```python
from build123d import *

# Parameters (mm, degrees)
AUFSATZ_LINEAR_AUSTRAGEN1_DEPTH = 5
SKIZZE2_W                       = 6
SKIZZE2_H                       = 10
AUFSATZ_LINEAR_AUSTRAGEN2_DEPTH = 10
FASE1_SIZE                      = 10
SKIZZE3_R                       = 1.6
SCHNITT_LINEAR_AUSTRAGEN1_DEPTH = 42
SKIZZE4_W                       = 42
SKIZZE4_H                       = 4
AUFSATZ_LINEAR_AUSTRAGEN3_DEPTH = 20
KREISMUSTER1_COUNT              = 3
VERRUNDUNG1_START               = -21
VERRUNDUNG1_DEPTH               = 6
VERRUNDUNG1_START_2             = 15
VERRUNDUNG1_2_DEPTH             = 6
VERRUNDUNG1_3_DEPTH             = 6
VERRUNDUNG1_4_DEPTH             = 6
VERRUNDUNG1_5_DEPTH             = 6
VERRUNDUNG1_6_DEPTH             = 6
VERRUNDUNG1_START_3             = -22
VERRUNDUNG1_7_DEPTH             = 44
VERRUNDUNG1_8_DEPTH             = 44
VERRUNDUNG1_9_DEPTH             = 44


with BuildPart() as part:
    # Skizze1 → Aufsatz-Linear austragen1 (new body)
    with BuildSketch(Plane(origin=(0, 0, 0), x_dir=(1, 0, 0), z_dir=(0, 1, 0))):
        with BuildLine():
            Line((93.122718948, -36.443918776), (41.161194721, -6.443918776))
            Line((41.161194721, -6.443918776), (26.161194721, -32.42468089))
            Line((26.161194721, -32.42468089), (78.122718948, -62.42468089))
            ThreePointArc((78.122718948, -62.42468089), (0, -100), (-78.122718948, -62.42468089))
            Line((-78.122718948, -62.42468089), (-26.161194721, -32.42468089))
            Line((-26.161194721, -32.42468089), (-41.161194721, -6.443918776))
            Line((-41.161194721, -6.443918776), (-93.122718948, -36.443918776))
            ThreePointArc((-93.122718948, -36.443918776), (-86.602540378, 50), (-15, 98.868599666))
            Line((-15, 98.868599666), (-15, 38.868599666))
            Line((-15, 38.868599666), (15, 38.868599666))
            Line((15, 38.868599666), (15, 98.868599666))
            ThreePointArc((15, 98.868599666), (86.602540378, 50), (93.122718948, -36.443918776))
        make_face()
    extrude(amount=AUFSATZ_LINEAR_AUSTRAGEN1_DEPTH)

    # Skizze2 → Aufsatz-Linear austragen2 (add)
    with BuildSketch(Plane(origin=(0, 5, 0), x_dir=(1, 0, 0), z_dir=(0, 1, 0))):
        Polygon((49.821448758, -11.443918776), (52.821448758, -6.247766354), (44.161194721, -1.247766354), (41.161194721, -6.443918776), align=None)
        with Locations((-18, 43.868599666)):
            Rectangle(SKIZZE2_W, SKIZZE2_H)
        with Locations((18, 43.868599666)):
            Rectangle(SKIZZE2_W, SKIZZE2_H)
        Polygon((26.161194721, -32.42468089), (23.161194721, -37.620833313), (31.821448758, -42.620833313), (34.821448758, -37.42468089), align=None)
        Polygon((-34.821448758, -37.42468089), (-31.821448758, -42.620833313), (-23.161194721, -37.620833313), (-26.161194721, -32.42468089), align=None)
        Polygon((-41.161194721, -6.443918776), (-44.161194721, -1.247766354), (-52.821448758, -6.247766354), (-49.821448758, -11.443918776), align=None)
    extrude(amount=AUFSATZ_LINEAR_AUSTRAGEN2_DEPTH)

    # Fase1
    fase1_edges = [part.edges().sort_by_distance(p)[0] for p in [
        (-18, 5, -48.868599666),
        (18, 5, -48.868599666),
        (51.321448758, 5, 8.845842565),
        (33.321448758, 5, 40.022757101),
        (-33.321448758, 5, 40.022757101),
        (-51.321448758, 5, 8.845842565),
    ]]
    chamfer(fase1_edges, length=FASE1_SIZE - 0.0001)  # a hair under: the kernel refuses the full size

    # Skizze3 → Schnitt-Linear austragen1 (cut)
    with BuildSketch(Plane(origin=(10.5, 0, 18.186533479), x_dir=(0.8660254037844384, 0, -0.5000000000000007), z_dir=(0.5000000000000006, 0, 0.8660254037844383))):
        with Locations((-45.868599666, 10)):
            Circle(SKIZZE3_R)
    schnitt_linear_austragen1 = extrude(amount=-SCHNITT_LINEAR_AUSTRAGEN1_DEPTH, mode=Mode.SUBTRACT)

    # Skizze4 → Aufsatz-Linear austragen3 (add)
    with BuildSketch(Plane(origin=(0, 5, 0), x_dir=(1, 0, 0), z_dir=(0, 1, 0))):
        with BuildLine():
            Line((-93.122718948, -36.443918776), (-88.740384046, -33.913776541))
            ThreePointArc((-88.740384046, -33.913776541), (-82.27241336, 47.5), (-15, 93.808315196))
            Line((-15, 93.808315196), (-15, 98.868599666))
            ThreePointArc((-15, 98.868599666), (-86.602540378, 50), (-93.122718948, -36.443918776))
        make_face()
        with BuildLine():
            Line((-78.122718948, -62.42468089), (-73.740384046, -59.894538655))
            ThreePointArc((-73.740384046, -59.894538655), (0, -95), (73.740384046, -59.894538655))
            Line((73.740384046, -59.894538655), (78.122718948, -62.42468089))
            ThreePointArc((78.122718948, -62.42468089), (0, -100), (-78.122718948, -62.42468089))
        make_face()
        with BuildLine():
            Line((93.122718948, -36.443918776), (88.740384046, -33.913776541))
            ThreePointArc((88.740384046, -33.913776541), (82.27241336, 47.5), (15, 93.808315196))
            Line((15, 93.808315196), (15, 98.868599666))
            ThreePointArc((15, 98.868599666), (86.602540378, 50), (93.122718948, -36.443918776))
        make_face()
        Polygon((-44.161194721, -1.247766354), (-23.161194721, -37.620833313), (-19.697093106, -35.620833313), (-40.697093106, 0.752233646), align=None)
        with Locations((0, 36.868599666)):
            Rectangle(SKIZZE4_W, SKIZZE4_H)
        Polygon((19.697093106, -35.620833313), (40.697093106, 0.752233646), (44.161194721, -1.247766354), (23.161194721, -37.620833313), align=None)
    extrude(amount=AUFSATZ_LINEAR_AUSTRAGEN3_DEPTH)

    # Kreismuster1: Schnitt-Linear austragen1 ×3 about axis
    kreismuster1_axis = Axis((0, 5, 0), (0, -1, 0))
    for i in range(1, KREISMUSTER1_COUNT):
        add(schnitt_linear_austragen1.rotate(kreismuster1_axis, i * 360 / KREISMUSTER1_COUNT), mode=Mode.SUBTRACT)

    # Verrundung1: read off the stored shape, not the designer's step
    # Verrundung1 outline → Verrundung1 (add)
    with BuildSketch(Plane.YZ.offset(VERRUNDUNG1_START)):
        with BuildLine():
            ThreePointArc((15, -39.868599666), (15.292893219, -39.161492885), (16, -38.868599666))
            Line((16, -38.868599666), (15, -38.868599666))
            Line((15, -38.868599666), (15, -39.868599666))
        make_face()
    extrude(amount=VERRUNDUNG1_DEPTH)

    # Verrundung1 2 outline → Verrundung1 2 (add)
    with BuildSketch(Plane.YZ.offset(VERRUNDUNG1_START_2)):
        with BuildLine():
            ThreePointArc((15, -39.868599666), (15.292893219, -39.161492885), (16, -38.868599666))
            Line((16, -38.868599666), (15, -38.868599666))
            Line((15, -38.868599666), (15, -39.868599666))
        make_face()
    extrude(amount=VERRUNDUNG1_2_DEPTH)

    # Verrundung1 3 outline → Verrundung1 3 (add)
    with BuildSketch(Plane(origin=(0, 0, 0), x_dir=(0.8660254037844386, 0, 0.4999999999999999), z_dir=(0.4999999999999999, 0, -0.8660254037844388)).offset(VERRUNDUNG1_START)):
        with BuildLine():
            Line((38.868599666, -15), (38.868599666, -16))
            ThreePointArc((38.868599666, -16), (39.161492885, -15.292893219), (39.868599666, -15))
            Line((39.868599666, -15), (38.868599666, -15))
        make_face()
    extrude(amount=VERRUNDUNG1_3_DEPTH)

    # Verrundung1 4 outline → Verrundung1 4 (add)
    with BuildSketch(Plane(origin=(0, 0, 0), x_dir=(0.8660254037844386, 0, 0.4999999999999999), z_dir=(0.4999999999999999, 0, -0.8660254037844388)).offset(VERRUNDUNG1_START_2)):
        with BuildLine():
            Line((38.868599666, -15), (38.868599666, -16))
            ThreePointArc((38.868599666, -16), (39.161492885, -15.292893219), (39.868599666, -15))
            Line((39.868599666, -15), (38.868599666, -15))
        make_face()
    extrude(amount=VERRUNDUNG1_4_DEPTH)

    # Verrundung1 5 outline → Verrundung1 5 (add)
    with BuildSketch(Plane(origin=(0, 0, 0), x_dir=(0.8660254037844384, 0, -0.5000000000000003), z_dir=(0.5000000000000003, 0, 0.8660254037844385)).offset(VERRUNDUNG1_START)):
        with BuildLine():
            Line((-38.868599666, 15), (-38.868599666, 16))
            ThreePointArc((-38.868599666, 16), (-39.161492885, 15.292893219), (-39.868599666, 15))
            Line((-39.868599666, 15), (-38.868599666, 15))
        make_face()
    extrude(amount=VERRUNDUNG1_5_DEPTH)

    # Verrundung1 6 outline → Verrundung1 6 (add)
    with BuildSketch(Plane(origin=(0, 0, 0), x_dir=(0.8660254037844384, 0, -0.5000000000000003), z_dir=(0.5000000000000003, 0, 0.8660254037844385)).offset(VERRUNDUNG1_START_2)):
        with BuildLine():
            Line((-38.868599666, 15), (-38.868599666, 16))
            ThreePointArc((-38.868599666, 16), (-39.161492885, 15.292893219), (-39.868599666, 15))
            Line((-39.868599666, 15), (-38.868599666, 15))
        make_face()
    extrude(amount=VERRUNDUNG1_6_DEPTH)

    # Verrundung1 7 outline → Verrundung1 7 (cut)
    with BuildSketch(Plane.YZ.offset(VERRUNDUNG1_START_3)):
        with BuildLine():
            Line((15, -48.868599666), (15, -47.211745417))
            ThreePointArc((15, -47.211745417), (14.69551813, -48.742479146), (13.828427125, -50.040172542))
            Line((13.828427125, -50.040172542), (15, -48.868599666))
        make_face()
    extrude(amount=VERRUNDUNG1_7_DEPTH, mode=Mode.SUBTRACT)

    # Verrundung1 8 outline → Verrundung1 8 (cut)
    with BuildSketch(Plane(origin=(0, 0, 0), x_dir=(0.8660254037844386, 0, 0.4999999999999999), z_dir=(0.4999999999999999, 0, -0.8660254037844388)).offset(VERRUNDUNG1_START_3)):
        with BuildLine():
            ThreePointArc((50.040172542, -13.828427125), (48.742479146, -14.69551813), (47.211745417, -15))
            Line((47.211745417, -15), (48.868599666, -15))
            Line((48.868599666, -15), (50.040172542, -13.828427125))
        make_face()
    extrude(amount=VERRUNDUNG1_8_DEPTH, mode=Mode.SUBTRACT)

    # Verrundung1 9 outline → Verrundung1 9 (cut)
    with BuildSketch(Plane(origin=(0, 0, 0), x_dir=(0.8660254037844384, 0, -0.5000000000000003), z_dir=(0.5000000000000003, 0, 0.8660254037844385)).offset(VERRUNDUNG1_START_3)):
        with BuildLine():
            ThreePointArc((-50.040172542, 13.828427125), (-48.742479146, 14.69551813), (-47.211745417, 15))
            Line((-47.211745417, 15), (-48.868599666, 15))
            Line((-48.868599666, 15), (-50.040172542, 13.828427125))
        make_face()
    extrude(amount=VERRUNDUNG1_9_DEPTH, mode=Mode.SUBTRACT)


solid = part.part
```
Verification items for the finished model (mm, model axes). A direction names the side the tool comes from. Coordinates: 2 decimals unless noted, no trailing zeros. Loops run counter-clockwise (first coordinate to the right, second up) from the corner with the lowest first, then second, coordinate; pieces in that order, holes last. Notation, with made-up numbers: (-6.75, 48.25) -> (36.25, 48.25) arc R30 cw to (36.25, 71.25) -> close; hole circle Ø4 at (25, -17.5). An arc over 180 degrees is marked (long way). Put each result on its own line as item: value.
1. Section check C-C, the plane x = 10.5. Record the boundary of the cut face in (y, z), then the cut area to 3 significant figures.
Result set:
outline: (0, -38.87) -> (25, -38.87) -> (25, -34.87) -> (5, -34.87) -> (5, 94.42) -> (25, 94.42) -> (25, 99.45) -> (0, 99.45) -> close
area: 872 mm^2
2. Section check B-B, the plane z = 25. Record the boundary of the cut face in (x, y).
Result set:
outline: (-96.82, 0) -> (-73.3, 0) -> (-73.3, 5) -> (-91.65, 5) -> (-91.65, 25) -> (-96.82, 25) -> close; (-30.45, 0) -> (30.45, 0) -> (30.45, 25) -> (25.83, 25) -> (25.83, 5) -> (-25.83, 5) -> (-25.83, 25) -> (-30.45, 25) -> close; (73.3, 0) -> (96.82, 0) -> (96.82, 25) -> (91.65, 25) -> (91.65, 5) -> (73.3, 5) -> close
3. Section check A-A, the plane x = 64. Record the boundary of the cut face in (y, z), then the cut area to 3 significant figures.
Result set:
outline: (0, -76.84) -> (25, -76.84) -> (25, -70.21) -> (5, -70.21) -> (5, 19.63) -> (0, 19.63) -> close; (0, 54.27) -> (5, 54.27) -> (5, 70.21) -> (25, 70.21) -> (25, 76.84) -> (0, 76.84) -> close
area: 860 mm^2
4. Gauge pin test, flat ends, axial feed: P1, Ø10, axis at x = -47, z = 8.5, coming from the +Y side; P2, Ø10, axis at x = 60, y = 10, coming from the -Z side; P3, Ø6, axis at y = 15, z = 24.5, coming from the +X side. Record the tip position at first contact, or that the pin passes through.
Result set:
P1: stops at y = 15
P2: stops at z = -83.52
P3: stops at x = 97.66
5. Thickness scan on line 1 (X direction, y = 16.5, z = 22.5); line 2 (Z direction, x = -3, y = 16.75); line 3 (Z direction, x = 29, y = 18.75). Record the ranges inside material, lowest first.
Result set:
line 1: x = -97.44 to -92.3, -31.89 to -27.27, 27.27 to 31.89, 92.3 to 97.44
line 2: z = -38.87 to -34.87, 94.95 to 99.95
line 3: z = -95.7 to -90.47, 19.51 to 27.51, 90.47 to 95.7
6. Section check D-D, the plane z = 79. Record the boundary of the cut face in (x, y), then the cut area to 3 significant figures.
Result set:
outline: (-61.31, 0) -> (61.31, 0) -> (61.31, 25) -> (52.76, 25) -> (52.76, 5) -> (-52.76, 5) -> (-52.76, 25) -> (-61.31, 25) -> close
area: 955 mm^2
7. Tool access check on faces 1 (the face through (31.844, 9.026, 39.121)), 2 (the face through (15, 4, -68)), 3 (the face through (-32, 25, 20)), 4 (the face through (-1.182, 14.86, 94.993)), 5 (the face through (33.2, 14.69, 40)). Record the directions out of +Z, -Z, +X, -X, +Y, -Y that give a thin tool (end or side, any length) a straight path to the whole face; none if there is none.
Result set:
face 1: none
face 2: -Z, +Y, -Y
face 3: +Z, -Z, +X, -X, +Y
face 4: +Y
face 5: +X, +Y
8. Mould release check, pull along X, two halves, no side actions. Record for faces 6 (the face through (-18, 15, -44)), 7 (the face through (-33.24, 14.69, 39.93)), 8 (the face through (-31.003, 8.438, 38.733)), 9 (the face through (38.08, 9.48, 42.82)): pulls with the +X half, pulls with the -X half, needs draft (parallel to the pull), parting line crosses it, or undercut.
Result set:
face 6: undercut
face 7: pulls with the -X half
face 8: undercut
face 9: pulls with the +X half
